```python
from build123d import *

# Parameters (mm, degrees)
F1_DEPTH = 127
F2_R     = 4
F2_W     = 20
F2_H     = 25.4
F3_DEPTH = 25


with BuildPart() as f1:
    # F0 (on Top) → F1 (new body)
    with BuildSketch(Plane.XY):
        Polygon((-13.266638, 11.597826), (-18.266638, 11.597826), (-18.266638, -13.402174), (6.733362, -13.402174), (6.733362, -8.402174), (-13.266638, -8.402174), align=None)
    extrude(amount=F1_DEPTH)

    # F2 (on face) → F3 (cut)
    with BuildSketch(Plane.XZ.offset(13.402174)):
        with Locations((-5.766638, 76.2)):
            Circle(F2_R)
        with Locations((-5.766638, 50.8)):
            Circle(F2_R)
        with Locations((-5.766638, 25.4)):
            Circle(F2_R)
        with Locations((-3.266638, 114.3)):
            Rectangle(F2_W, F2_H)
    extrude(amount=-F3_DEPTH, mode=Mode.SUBTRACT)


solid = f1.part
```
Check sheet for the modelled part. Datum: model origin and axes. Units: mm. A direction names the side the tool comes from. Give positions to 0.01 mm unless a question says otherwise; leave off trailing zeros. Write each loop counter-clockwise with the first axis right and the second up, starting at its lowest first coordinate (ties: lowest second). Pieces come first, ordered by that corner, then holes. Notation, with made-up numbers: (58, -20.75) -> (68, -20.75) arc R14 cw to (68, -5.75) -> close; hole circle Ø3 at (34, -32.75). An arc over 180 degrees is marked (long way). Use CSV: the item, a comma, the result in double quotes. Start each with the question number.
Q1. Cross-section at A-A on z = 76.2. Enter the section's corners in (x, y).
Q2. Cross-section at B-B on x = -6. Enter the section's corners in (y, z), and give its area (3 significant figures).
Q3. Cross-section at D-D on y = -0.25. Enter the section's corners in (x, z).
Q4. Depth check by flat-ended pin: P1, Ø13, axis at x = -5.77, z = 76.2, coming from the +Y side; P2, Ø7, axis at x = -5.77, z = 50.8, coming from the +Y side; P3, Ø1, axis at y = 3.5, z = 78.5, coming from the +X side; P4, Ø4, axis at x = 0, y = -10, coming from the +Z side. Enter the tip coordinate at first touch or a pass-through.
Q5. Tool access check on faces 1 (the flat face through (-1, -8.402, 50)), 2 (the flat face through (-3, -11, 101.6)), 3 (the flat face through (-18.267, -1, 63)). Record the directions out of +Z, -Z, +X, -X, +Y, -Y that give a thin tool (end or side, any length) a straight path to the whole face; none if there is none.
Q6. Release check for a two-part mould opening along X. For faces 4 (the cylindrical face through (-3.92, -10.94, 72.65)), 5 (the flat face through (6.733, -11, 50)), 6 (the flat face through (-11, -13.402, 48)) record: +X half, -X half, draft (parallel to the pull), parting line (faces both ways), or undercut.
Q7. Scan lines: line 1 along Y through (x, z) = (2.25, 8.5); line 2 along X through (y, z) = (-4.5, 91); line 3 along Z through (x, y) = (3, -10.5). Record each from-to range of solid material in increasing order.
Q8. Cross-section at C-C on z = 38. Enter the section's corners in (x, y), and give its area (3 significant figures).
Working result:
1,outline,"(-18.27, -13.4) -> (-9.77, -13.4) -> (-9.77, -8.4) -> (-13.27, -8.4) -> (-13.27, 11.6) -> (-18.27, 11.6) -> close; (-1.77, -13.4) -> (6.73, -13.4) -> (6.73, -8.4) -> (-1.77, -8.4) -> close"
2,outline,"(-13.4, 0) -> (-8.4, 0) -> (-8.4, 21.41) -> (-13.4, 21.41) -> close; (-13.4, 29.39) -> (-8.4, 29.39) -> (-8.4, 46.81) -> (-13.4, 46.81) -> close; (-13.4, 54.79) -> (-8.4, 54.79) -> (-8.4, 72.21) -> (-13.4, 72.21) -> close; (-13.4, 80.19) -> (-8.4, 80.19) -> (-8.4, 101.6) -> (-13.4, 101.6) -> close"
2,area,"388 mm^2"
3,outline,"(-18.27, 0) -> (-13.27, 0) -> (-13.27, 127) -> (-18.27, 127) -> close"
4,P1,"stops at y = -8.4"
4,P2,"passes through"
4,P3,"stops at x = -13.27"
4,P4,"stops at z = 101.6"
5,face 1,"+Z, -Z, +X, +Y"
5,face 2,"+Z, +X, +Y, -Y"
5,face 3,"+Z, -Z, -X, +Y, -Y"
6,face 4,"undercut"
6,face 5,"+X half"
6,face 6,"draft"
7,line 1,"y = -13.4 to -8.4"
7,line 2,"x = -18.27 to -13.27"
7,line 3,"z = 0 to 101.6"
8,outline,"(-18.27, -13.4) -> (6.73, -13.4) -> (6.73, -8.4) -> (-13.27, -8.4) -> (-13.27, 11.6) -> (-18.27, 11.6) -> close"
8,area,"225 mm^2"
